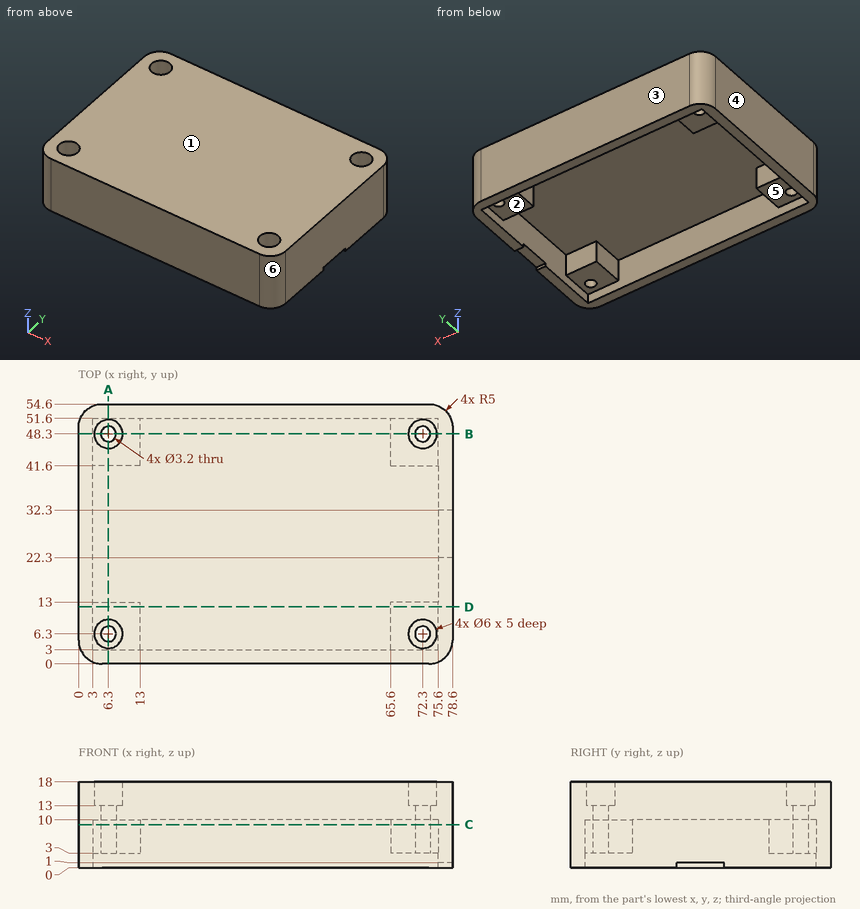
Geometry check sheet. Reference: drawing and pictorial views, mm from the part's lowest x, y, z. A direction names the side the tool comes from. Round coordinates to 2 decimals unless told otherwise and drop trailing zeros. Order: outer loops, then holes, each group sorted by start corner. A loop starts at its lowest first (then second) coordinate and runs counter-clockwise, first axis right, second up. Notation, with made-up numbers: (8, -21.5) - (21, -21.5) arc R30 ccw to (21, 4.5) - close; hole circle Ø11 at (60.5, 56). An arc over 180 degrees is marked (long way). Use a Markdown table: item, result. Add a question column.
1) Section check D-D (y = 12). Record the cut outline in (x, z).
2) Mould release check, pull along X, two halves, no side actions. Record for the marked faces 3, 4, 5 and 6: released by +X, released by -X, zero draft, split by the parting line, or undercut.
3) Thickness scan on line 1 along Y through (x, z) = (6.3, 16.95); line 2 along Y through (x, z) = (6.3, 5.75); line 3 along Y through (x, z) = (31.5, 3). Record the ranges inside material, lowest first.
4) Set-up check for the marked faces 1 and 2: record each of +Z, -Z, +X, -X, +Y, -Y from which the full face is reachable in a straight line by a thin tool's end or side.
5) Section check B-B (y = 48.3). Record the cut outline in (x, z).
6) Gauge pin test, flat ends, axial feed: P1, Ø1.5, axis at x = 14.5, z = 13.5, coming from the -Y side; P2, Ø11, axis at x = 68.5, y = 10, coming from the -Z side; P3, Ø1.9, axis at x = 72.3, y = 6.3, coming from the +Z side; P4, Ø6, axis at x = 68.5, y = 23, coming from the -Z side. Record the tip position at first contact, or that the pin passes through.
7) Section check C-C (z = 9). Record the cut outline in (x, y).
8) Section check A-A (x = 6.3). Record the cut outline in (y, z), then the cut area to 3 significant figures.
Established:
| question | item | result |
|---|---|---|
| 1 | outline | (0, 0) - (3, 0) - (3, 3) - (13, 3) - (13, 10) - (65.6, 10) - (65.6, 3) - (75.6, 3) - (75.6, 0) - (78.6, 0) - (78.6, 18) - (0, 18) - close |
| 2 | face 3 | zero draft |
| 2 | face 4 | released by -X |
| 2 | face 5 | undercut |
| 2 | face 6 | released by +X |
| 3 | line 1 | 0 to 3.3, 9.3 to 45.3, 51.3 to 54.6 |
| 3 | line 2 | 0 to 4.7, 7.9 to 13, 41.6 to 46.7, 49.9 to 54.6 |
| 3 | line 3 | 0 to 3, 51.6 to 54.6 |
| 4 | face 1 | +Z, +X, -X, +Y, -Y |
| 4 | face 2 | -Z |
| 5 | outline | (0, 0) - (3, 0) - (3, 3) - (4.7, 3) - (4.7, 13) - (3.3, 13) - (3.3, 18) - (0, 18) - close; (7.9, 3) - (13, 3) - (13, 10) - (65.6, 10) - (65.6, 3) - (70.7, 3) - (70.7, 13) - (69.3, 13) - (69.3, 18) - (9.3, 18) - (9.3, 13) - (7.9, 13) - close; (73.9, 3) - (75.6, 3) - (75.6, 0) - (78.6, 0) - (78.6, 18) - (75.3, 18) - (75.3, 13) - (73.9, 13) - close |
| 6 | P1 | y = 0 |
| 6 | P2 | z = 3 |
| 6 | P3 | through |
| 6 | P4 | z = 10 |
| 7 | outline | (0, 5) arc R5 ccw to (5, 0) - (73.6, 0) arc R5 ccw to (78.6, 5) - (78.6, 49.6) arc R5 ccw to (73.6, 54.6) - (5, 54.6) arc R5 ccw to (0, 49.6) - close; hole (3, 13) - (13, 13) - (13, 3) - (65.6, 3) - (65.6, 13) - (75.6, 13) - (75.6, 41.6) - (65.6, 41.6) - (65.6, 51.6) - (13, 51.6) - (13, 41.6) - (3, 41.6) - close; hole circle Ø3.2 at (6.3, 6.3); hole circle Ø3.2 at (6.3, 48.3); hole circle Ø3.2 at (72.3, 6.3); hole circle Ø3.2 at (72.3, 48.3) |
| 8 | outline | (0, 0) - (3, 0) - (3, 3) - (4.7, 3) - (4.7, 13) - (3.3, 13) - (3.3, 18) - (0, 18) - close; (7.9, 3) - (13, 3) - (13, 10) - (41.6, 10) - (41.6, 3) - (46.7, 3) - (46.7, 13) - (45.3, 13) - (45.3, 18) - (9.3, 18) - (9.3, 13) - (7.9, 13) - close; (49.9, 3) - (51.6, 3) - (51.6, 0) - (54.6, 0) - (54.6, 18) - (51.3, 18) - (51.3, 13) - (49.9, 13) - close |
| 8 | area | 513 mm2 |
